Check sheet for the modelled part. Datum: model origin and axes. Units: mm. Face numbers are marked on the shaded views. A direction names the side the tool comes from. Round coordinates to 2 decimals unless told otherwise and drop trailing zeros. Write each loop counter-clockwise with the first axis right and the second up, starting at its lowest first coordinate (ties: lowest second). Pieces come first, ordered by that corner, then holes.
Item 1: Cross-section at C-C on x = -110. Enter the section's corners in (y, z), plus the area to 3 significant figures.
Item 2: Cross-section at B-B on y = 0.5. Enter the section's corners in (x, z), plus the area to 3 significant figures.
Item 3: Release check for a two-part mould opening along X. For the marked faces 6, 7 and 8 record: +X half, -X half, draft (parallel to the pull), parting line (faces both ways), or undercut.
Item 4: Cross-section at D-D on x = 0. Enter the section's corners in (y, z).
Item 5: Go/stop test with flat-tipped pins: pin 1 Ø12.5 at (x, y) = (-112.5, 13.5) entering from +Z; pin 2 Ø1 at (x, y) = (-64.5, -3) entering from -Z; pin 3 Ø20 at (x, y) = (-110, 18) entering from -Z; pin 4 Ø11 at (x, y) = (-110, 17.5) entering from +Z. Record where each tip stops, or that it passes through.
Item 6: Cross-section at A-A on z = 0. Enter the section's corners in (x, y).
Item 7: Material ranges on line 1 (X direction, y = 9.5, z = 0); line 2 (Y direction, x = -110, z = 9); line 3 (X direction, y = 2.5, z = 0), recorded low to high.
Item 8: Tool access check on the marked faces 1, 2, 3, 4 and 5. Record the directions out of +Z, -Z, +X, -X, +Y, -Y that give a thin tool (end or side, any length) a straight path to the whole face; none if there is none.
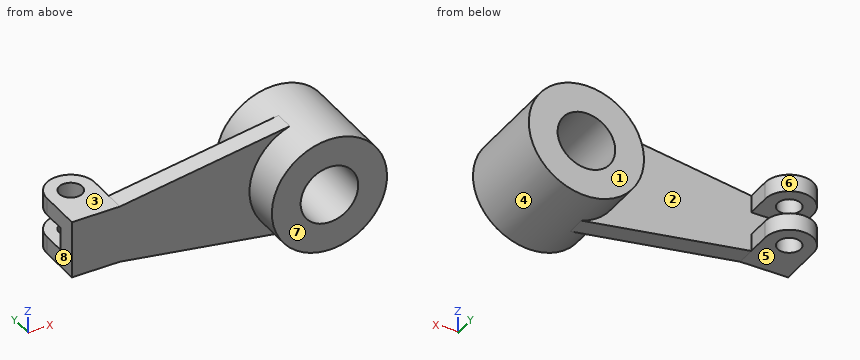
from build123d import *

# Parameters (mm, degrees)
SKETCH1_R           = 30
SKETCH1_R_2         = 15
BOSS_EXTRUDE2_DEPTH = 25
BOSS_EXTRUDE3_DEPTH = 5
BOSS_EXTRUDE5_DEPTH = 9
SKETCH6_R           = 6
BOSS_EXTRUDE6_DEPTH = 9
SKETCH7_R           = 6
CUT_EXTRUDE2_DEPTH  = 46


with BuildPart() as part:
    # Sketch1 → Boss-Extrude2 (new body, symmetric)
    with BuildSketch(Plane(origin=(0, 0, 0), x_dir=(1, 0, 0), z_dir=(0, 1, 0))):
        with Locations(Location((0, 0, 0), (0, 0, 270))):  # turned: the seam where the file's is
            Circle(SKETCH1_R)
        with Locations(Location((0, 0, 0), (0, 0, 270))):  # turned: the seam where the file's is
            Circle(SKETCH1_R_2, mode=Mode.SUBTRACT)
    extrude(amount=BOSS_EXTRUDE2_DEPTH, both=True)

    # Sketch3 → Boss-Extrude3 (add, symmetric)
    with BuildSketch(Plane(origin=(0, 0, 0), x_dir=(1, 0, 0), z_dir=(0, 1, 0))):
        with BuildLine():
            Line((-97.5, 15), (-122.5, 15))
            Line((-122.5, 15), (-122.5, -15))
            Line((-122.5, -15), (-97.5, -15))
            Line((-97.5, -15), (-9.01734104, -28.612716763))
            ThreePointArc((-9.01734104, -28.612716763), (-30, 0), (-9.01734104, 28.612716763))
            Line((-9.01734104, 28.612716763), (-97.5, 15))
        make_face()
    extrude(amount=BOSS_EXTRUDE3_DEPTH, both=True)

    # Sketch4 → Boss-Extrude5 (add)
    with BuildSketch(Plane.XY.offset(15)):
        with BuildLine():
            Line((-122.5, 5), (-122.5, 17.5))
            ThreePointArc((-122.5, 17.5), (-110, 30), (-97.5, 17.5))
            Line((-97.5, 17.5), (-97.5, 5))
            Line((-97.5, 5), (-97.5, -5))
            Line((-97.5, -5), (-122.5, -5))
            Line((-122.5, -5), (-122.5, 5))
        make_face()
    extrude(amount=-BOSS_EXTRUDE5_DEPTH)

    # Sketch6 → Boss-Extrude6 (add)
    with BuildSketch(Plane(origin=(0, 0, -15), x_dir=(-1, 0, 0), z_dir=(0, 0, -1))):
        with BuildLine():
            Line((97.5, 5), (97.5, 17.5))
            ThreePointArc((97.5, 17.5), (110, 30), (122.5, 17.5))
            Line((122.5, 17.5), (122.5, 5))
            Line((122.5, 5), (122.5, -5))
            Line((122.5, -5), (97.5, -5))
            Line((97.5, -5), (97.5, 5))
        make_face()
        with Locations((110, 17.5)):
            Circle(SKETCH6_R, mode=Mode.SUBTRACT)
    extrude(amount=-BOSS_EXTRUDE6_DEPTH)

    # Sketch7 → Cut-Extrude2 (cut, through all)
    with BuildSketch(Plane.XY.offset(15)):
        with Locations(Location((-110, 17.5, 0), (0, 0, 180))):  # turned: the seam where the file's is
            Circle(SKETCH7_R)
    extrude(amount=-CUT_EXTRUDE2_DEPTH, mode=Mode.SUBTRACT)


solid = part.part
Response values:
1. outline: (-5, -15) - (11.5, -15) - (11.5, -6) - (5, -6) - (5, 6) - (11.5, 6) - (11.5, 15) - (-5, 15) - close; (23.5, -15) - (30, -15) - (30, -6) - (23.5, -6) - close; (23.5, 6) - (30, 6) - (30, 15) - (23.5, 15) - close
1. area: 534 mm2
2. outline: (-122.5, -15) - (-97.5, -15) - (-9.02, -28.61) arc R30 ccw (long way) to (-9.02, 28.61) - (-97.5, 15) - (-122.5, 15) - close; hole circle Ø30 at (0, 0)
2. area: 5,850 mm2
3. face 6: undercut
3. face 7: draft
3. face 8: -X half
4. outline: (-25, -30) - (25, -30) - (25, -15) - (-25, -15) - close; (-25, 15) - (25, 15) - (25, 30) - (-25, 30) - close
5. pin 1: stops at z = 15
5. pin 2: stops at z = -20.15
5. pin 3: stops at z = -15
5. pin 4: passes through
6. outline: (-122.5, -5) - (-30, -5) - (-30, -25) - (-15, -25) - (-15, 25) - (-30, 25) - (-30, 5) - (-122.5, 5) - close; (15, -25) - (30, -25) - (30, 25) - (15, 25) - close
7. line 1: x = -30 to -15, 15 to 30
7. line 2: y = -5 to 11.5, 23.5 to 30
7. line 3: x = -122.5 to -15, 15 to 30
8. face 1: +Z, -Z, +X, +Y
8. face 2: +Y
8. face 3: +Z, -X, +Y, -Y
8. face 4: none
8. face 5: -Z, -X, +Y, -Y
